from build123d import *

# Parameters (mm, degrees)
SKETCH1_W           = 112
SKETCH1_H           = 88.5
BOSS_EXTRUDE1_DEPTH = 3
SKETCH2_R           = 1.1
CUT_EXTRUDE1_DEPTH  = 72.435722856
SKETCH3_W           = 112
SKETCH3_H           = 88.5
SKETCH3_W_2         = 111.6
SKETCH3_H_2         = 88.1
CUT_EXTRUDE2_DEPTH  = 72.435722856
SKETCH4_R           = 2.25
CUT_EXTRUDE3_DEPTH  = 2


with BuildPart() as part:
    # Sketch1 → Boss-Extrude1 (new body)
    with BuildSketch(Plane.XY):
        Rectangle(SKETCH1_W, SKETCH1_H)
    extrude(amount=BOSS_EXTRUDE1_DEPTH)

    # Sketch2 → Cut-Extrude1 (cut, through all)
    with BuildSketch(Plane.XY.offset(3)):
        with Locations((-53, 41.25)):
            Circle(SKETCH2_R)
        with Locations((53, 41.25)):
            Circle(SKETCH2_R)
        with Locations((53, -41.25)):
            Circle(SKETCH2_R)
        with Locations((-53, -41.25)):
            Circle(SKETCH2_R)
    extrude(amount=-CUT_EXTRUDE1_DEPTH, mode=Mode.SUBTRACT)

    # Sketch3 → Cut-Extrude2 (cut, through all)
    with BuildSketch(Plane.XY.offset(3)):
        Rectangle(SKETCH3_W, SKETCH3_H)
        Rectangle(SKETCH3_W_2, SKETCH3_H_2, mode=Mode.SUBTRACT)
    extrude(amount=-CUT_EXTRUDE2_DEPTH, mode=Mode.SUBTRACT)

    # Sketch4 → Cut-Extrude3 (cut)
    with BuildSketch(Plane.XY.offset(3)):
        with Locations((-53, 41.25)):
            Circle(SKETCH4_R)
        with Locations((53, 41.25)):
            Circle(SKETCH4_R)
        with Locations((53, -41.25)):
            Circle(SKETCH4_R)
        with Locations((-53, -41.25)):
            Circle(SKETCH4_R)
    extrude(amount=-CUT_EXTRUDE3_DEPTH, mode=Mode.SUBTRACT)


solid = part.part
Design review of the part built by this model. Coordinates are the model's own, in mm. A direction names the side the tool comes from. Give positions to 0.01 mm unless a question says otherwise; leave off trailing zeros. Use CSV: the item, a comma, the result in double quotes. Start each with the question number.
1. Insertion check: P1, Ø3.5, axis at x = 53, y = 41.25, coming from the +Z side; P2, Ø2, axis at x = 53, y = -41.25, coming from the +Z side. Each pin has a flat end and moves straight along its axis. Give the tip position at first contact, or say it passes through.
2. Draft analysis for pull direction Y (two halves, no side actions). For faces 3 (the flat face through (-55.8, -1, 2)), 4 (the cylindrical face through (-53.811, 41.993, 0.507)), 5 (the flat face through (-1, 44.05, 2)), 6 (the flat face through (-1, -44.05, 2)), state which applies: released by +Y, released by -Y, zero draft, split by the parting line, or undercut.
3. Machinability: for faces 1 (the cylindrical face through (-53.811, -40.507, 0.507)), 2 (the flat face through (-54, -40, 1)), which of the approach directions +Z, -Z, +X, -X, +Y, -Y give a long, thin tool a straight path to every point of the face, cutting with its end or side? Answer none if there is none.
4. Wall thickness on L1, parallel to Y at x = 53, z = 0.65; L2, parallel to Y at x = -53, z = 2.25: over which ranges is each line inside the solid? List them lowest first.
Results found:
1,P1,"stops at z = 1"
1,P2,"passes through"
2,face 3,"zero draft"
2,face 4,"undercut"
2,face 5,"released by +Y"
2,face 6,"released by -Y"
3,face 1,"+Z, -Z"
3,face 2,"+Z"
4,L1,"y = -44.05 to -42.35, -40.15 to 40.15, 42.35 to 44.05"
4,L2,"y = -44.05 to -43.5, -39 to 39, 43.5 to 44.05"
